Here's the drawing with two shaded views (mm, measured from the low corner). I have some questions. A direction names the side the tool comes from. Coordinates: 2 decimals unless noted, no trailing zeros. Loops run counter-clockwise (first coordinate to the right, second up) from the corner with the lowest first, then second, coordinate; pieces in that order, holes last.
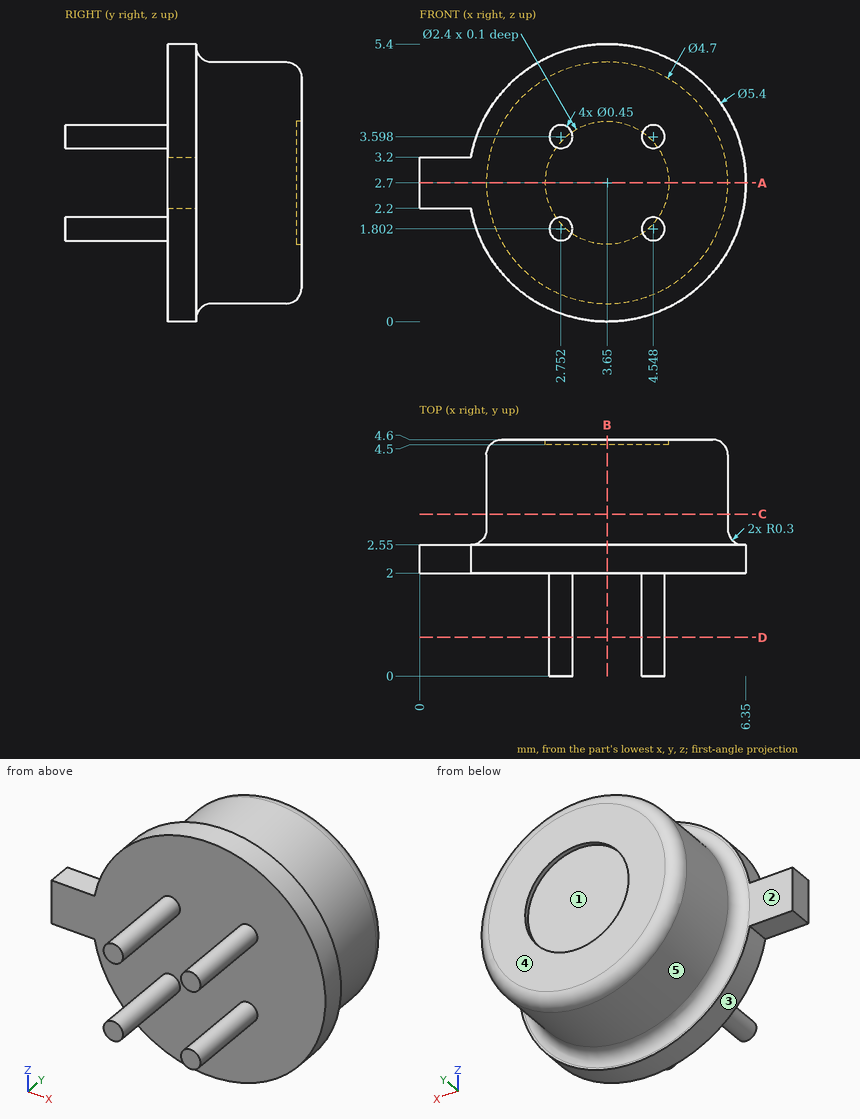
(1) I want a section at C-C on y = 3.15. Write out the boundary of the cut face in (x, z).
Check values:
outline: circle Ø4.7 at (3.65, 2.7)
(2) Which directions (+Z, -Z, +X, -X, +Y, -Y) give clear straight access to the entire face, cutting with the end or side of a thin tool? Please do the marked faces 4 and 5.
Check values:
face 4: +Z, -Z, +X, -X, +Y
face 5: +Y
(3) I want a section at B-B on x = 3.65. Write out the boundary of the cut face in (y, z), then the cut area to 3 significant figures.
Check values:
outline: (2, 0) - (2.55, 0) - (2.55, 0.05) arc R0.3 cw to (2.85, 0.35) - (4.3, 0.35) arc R0.3 ccw to (4.6, 0.65) - (4.6, 1.5) - (4.5, 1.5) - (4.5, 3.9) - (4.6, 3.9) - (4.6, 4.75) arc R0.3 ccw to (4.3, 5.05) - (2.85, 5.05) arc R0.3 cw to (2.55, 5.35) - (2.55, 5.4) - (2, 5.4) - close
area: 12.4 mm2
(4) If I drill on probe 1 along Y at (x, z) = (2, 1.8); probe 2 along Y at (x, z) = (4, 3.3); probe 3 along X at (y, z) = (2.75, 1.9), over which ranges is the centre line in solid material (lowest first)?
Check values:
probe 1: y = 2 to 4.6
probe 2: y = 2 to 4.5
probe 3: x = 1.42 to 5.88
(5) I'm going to push flat-ended pins straight in: pin 1 (0.6 mm diameter, centred on x = 0.5, y = 2.5, fed in from -Z); pin 2 (2 mm diameter, centred on x = 3.65, z = 2.7, fed in from +Y); pin 3 (0.6 mm diameter, centred on x = 0.5, y = 2.5, fed in from +Z). Where does each tip first touch, or does it pass through?
Check values:
pin 1: stops at z = 2.2
pin 2: stops at y = 4.5
pin 3: stops at z = 3.2
(6) If we mould it in two halves opening along Z, with no side actions, what happens to the marked faces 1, 2 and 3? For each: released by +Z, released by -Z, zero draft, split by the parting line, or undercut.
Check values:
face 1: undercut
face 2: zero draft
face 3: split by the parting line
(7) I want a section at D-D on y = 0.75. Write out the boundary of the cut face in (x, z) (3 decimals).
Check values:
outline: circle Ø0.45 at (2.752, 1.802); circle Ø0.45 at (2.752, 3.598); circle Ø0.45 at (4.548, 1.802); circle Ø0.45 at (4.548, 3.598)
(8) I want a section at A-A on z = 2.7. Write out the boundary of the cut face in (x, y).
Check values:
outline: (0, 2) - (6.35, 2) - (6.35, 2.55) - (6.3, 2.55) arc R0.3 cw to (6, 2.85) - (6, 4.3) arc R0.3 ccw to (5.7, 4.6) - (4.85, 4.6) - (4.85, 4.5) - (2.45, 4.5) - (2.45, 4.6) - (1.6, 4.6) arc R0.3 ccw to (1.3, 4.3) - (1.3, 2.85) arc R0.3 cw to (1, 2.55) - (0, 2.55) - close
